```python
from build123d import *

# Parameters (mm, degrees)
EXTRUDE_1_DEPTH = 20
CHAMFER_1_SIZE  = 0.3
CHAMFER_1_SIZE2 = 0.261758731
CHAMFER_2_SIZE2 = 0.214216777
CHAMFER_2_SIZE  = 0.3
CHAMFER_3_SIZE  = 0.15


with BuildPart() as part:
    # Эскиз1 → Вытянуть1 (new body)
    with BuildSketch(Plane(origin=(0, 0, 0), x_dir=(1, 0, 0), z_dir=(0, 1, 0))):
        Polygon((0, 0), (11.982938249, 15.901896151), (0, 15.901896151), align=None)
    extrude(amount=EXTRUDE_1_DEPTH)

    # Фаска1
    chamfer_1_edges = [part.edges().sort_by_distance(p)[0] for p in [
        (0, 10, 0),
    ]]
    chamfer_1_side = [part.faces().sort_by_distance(p)[0] for p in [
        (0, 10, -7.950948075),
    ]]
    chamfer(chamfer_1_edges, length=CHAMFER_1_SIZE, length2=CHAMFER_1_SIZE2, reference=chamfer_1_side[0])

    # Фаска2
    chamfer_2_edges = [part.edges().sort_by_distance(p)[0] for p in [
        (11.982938249, 10, -15.901896151),
    ]]
    chamfer(chamfer_2_edges, length=CHAMFER_2_SIZE, length2=CHAMFER_2_SIZE2)

    # Фаска3
    chamfer_3_edges = [part.edges().sort_by_distance(p)[0] for p in [
        (5.884360736, 0, -15.901896151),
        (5.884360736, 20, -15.901896151),
        (0, 20, -8.100948075),
        (0, 0, -8.100948075),
        (0, 10, -15.901896151),
    ]]
    chamfer(chamfer_3_edges, length=CHAMFER_3_SIZE)


solid = part.part
```
Part model, mm, in its own coordinate system. Round coordinates to 2 decimals unless told otherwise and drop trailing zeros. Loops run counter-clockwise (first coordinate to the right, second up) from the corner with the lowest first, then second, coordinate; pieces in that order, holes last.
1. Drill centre lines: line 1 along Z through (x, y) = (2.5, 12.25); line 2 along X through (y, z) = (5.5, -7.5); line 3 along X through (y, z) = (14.75, -1). Where is each one in solid material? Low to high.
Solutions:
line 1: z = -15.9 to -3.32
line 2: x = 0 to 5.65
line 3: x = 0 to 0.75
2. Flat gauge pin, fed straight in: pin 1 (6 mm diameter, centred on x = 4.5, y = 5.5, fed in from +Z). Where does the tip first touch, or does it go through?
Solutions:
pin 1: stops at z = -1.99
3. Slice it at B-B (x = 10.25). Give the cut face in (y, z).
Solutions:
outline: (0, -15.75) - (0.15, -15.9) - (19.85, -15.9) - (20, -15.75) - (20, -13.6) - (0, -13.6) - close
4. Slice it at A-A (y = 13.5). Give the cut face in (x, z), and give its area (3 significant figures).
Solutions:
outline: (0, -15.75) - (0.15, -15.9) - (11.77, -15.9) - (11.8, -15.66) - (0.16, -0.21) - (0, -0.3) - close
area: 95.2 mm2
5. Two-plate mould, pull along Y, no slides. Class faces 1 (the face through (5.9, 9.86, -7.83)), 2 (the face through (5, 0, -10)), 3 (the face through (5, 20, -10)): pulls with the +Y half, pulls with the -Y half, needs draft (parallel to the pull), parting line crosses it, or undercut.
Solutions:
face 1: needs draft
face 2: pulls with the -Y half
face 3: pulls with the +Y half
